Could you check a few things on this model? Use its own coordinates, in mm. Face numbers are marked on the shaded views. A direction names the side the tool comes from. Round coordinates to 2 decimals unless told otherwise and drop trailing zeros. Loops run counter-clockwise (first coordinate to the right, second up) from the corner with the lowest first, then second, coordinate; pieces in that order, holes last. Notation, with made-up numbers: M -6.5,2 L 27.5,2 A22 cw 27.5,41 Z; hole C -2.5,-34.5 d3. An arc over 180 degrees is marked long. Answer in a Markdown table with one row per item.
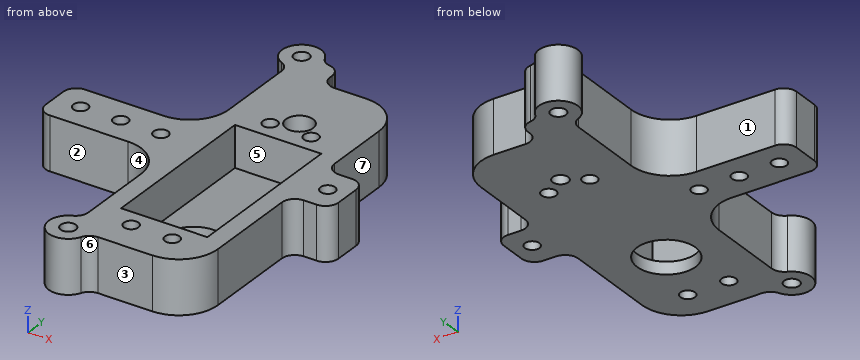
```python
from build123d import *

# Parameters (mm, degrees)
SKETCH1_W               = 31.75
SKETCH1_H               = 12.7
SKETCH1_W_2             = 30
SKETCH1_H_2             = 7
BOSS_EXTRUDE1_DEPTH     = 13
SKETCH4_R               = 1.778
CUT_EXTRUDE3_DEPTH      = 14
SKETCH5_W               = 21
SKETCH5_H               = 41
CUT_EXTRUDE4_DEPTH      = 10
SKETCH6_R               = 7.112
CUT_EXTRUDE5_DEPTH      = 4
SKETCH7_W               = 31.75
SKETCH7_H               = 12.7
CUT_EXTRUDE6_DEPTH      = 6.35
SKETCH10_R              = 1.905
CUT_EXTRUDE8_DEPTH      = 14
SKETCH11_R              = 3.302
CUT_EXTRUDE9_DEPTH      = 9.525
SKETCH13_W              = 9.525
SKETCH13_H              = 12.7
SKETCH13_R              = 1.778
BOSS_EXTRUDE2_DEPTH     = 13
BOSS_EXTRUDE3_DEPTH     = 13
SKETCH18_R              = 1.8415
CUT_EXTRUDE10_DEPTH     = 14
FILLET1_R               = 9.525
FILLET2_R               = 3.175
SKETCH19_W              = 22.225
SKETCH19_H              = 12.7
BOSS_EXTRUDE4_DEPTH     = 7.62
SKETCH8_R               = 1.778
CUT_EXTRUDE7_DEPTH      = 7.35
CUT_EXTRUDE7_DEPTH_BACK = 17.78
FILLET3_R               = 3.175


with BuildPart() as part:
    # Sketch1 → Boss-Extrude1 (new body)
    with BuildSketch(Plane.XY):
        Polygon((31.75, 12.7), (31.75, 0), (31.75, -28.65), (61.75, -28.65), (61.75, 0), (61.75, 12.7), (61.75, 41.35), (31.75, 41.35), align=None)
        with Locations((15.875, 6.35)):
            Rectangle(SKETCH1_W, SKETCH1_H)
        with Locations((46.75, -32.15)):
            Rectangle(SKETCH1_W_2, SKETCH1_H_2)
    extrude(amount=BOSS_EXTRUDE1_DEPTH)

    # Sketch4 → Cut-Extrude3 (cut, through all)
    with BuildSketch(Plane.XY.offset(13)):
        with Locations((41.75, 22.199999832)):
            Circle(SKETCH4_R)
        with Locations((51.75, 22.199999832)):
            Circle(SKETCH4_R)
        with Locations((41.75, -27.800000168)):
            Circle(SKETCH4_R)
        with Locations((51.75, -27.800000168)):
            Circle(SKETCH4_R)
    extrude(amount=-CUT_EXTRUDE3_DEPTH, mode=Mode.SUBTRACT)

    # Sketch5 → Cut-Extrude4 (cut)
    with BuildSketch(Plane.XY.offset(13)):
        with Locations((46.75, -2.800000024)):
            Rectangle(SKETCH5_W, SKETCH5_H)
    extrude(amount=-CUT_EXTRUDE4_DEPTH, mode=Mode.SUBTRACT)

    # Sketch6 → Cut-Extrude5 (cut, through all)
    with BuildSketch(Plane.XY.offset(3)):
        with Locations((46.75, -12.700000168)):
            Circle(SKETCH6_R)
    extrude(amount=-CUT_EXTRUDE5_DEPTH, mode=Mode.SUBTRACT)

    # Sketch7 → Cut-Extrude6 (cut)
    with BuildSketch(Plane(origin=(0, 0, 0), x_dir=(-1, 0, 0), z_dir=(0, 0, -1))):
        with Locations((-15.875, 6.35)):
            Rectangle(SKETCH7_W, SKETCH7_H)
    extrude(amount=-CUT_EXTRUDE6_DEPTH, mode=Mode.SUBTRACT)

    # Sketch10 → Cut-Extrude8 (cut, through all)
    with BuildSketch(Plane(origin=(0, 0, 0), x_dir=(-1, 0, 0), z_dir=(0, 0, -1))):
        with Locations((-46.75, 25.4)):
            Circle(SKETCH10_R)
    extrude(amount=-CUT_EXTRUDE8_DEPTH, mode=Mode.SUBTRACT)

    # Sketch11 → Cut-Extrude9 (cut)
    with BuildSketch(Plane.XY.offset(13)):
        with Locations((46.75, 25.4)):
            Circle(SKETCH11_R)
    extrude(amount=-CUT_EXTRUDE9_DEPTH, mode=Mode.SUBTRACT)

    # Sketch13 → Boss-Extrude2 (add)
    with BuildSketch(Plane.XY.offset(13)):
        with Locations((66.5125, 6.35)):
            Rectangle(SKETCH13_W, SKETCH13_H)
        with Locations((66.5125, 6.35)):
            Circle(SKETCH13_R, mode=Mode.SUBTRACT)
    extrude(amount=-BOSS_EXTRUDE2_DEPTH)

    # Sketch17 → Boss-Extrude3 (add)
    with BuildSketch(Plane.XY.offset(13)):
        with BuildLine():
            ThreePointArc((36.5125, 48.359214074), (28.382403955, 51.726810119), (31.75, 43.596714074))
            Line((31.75, 43.596714074), (31.75, 48.359214074))
            Line((31.75, 48.359214074), (36.5125, 48.359214074))
        make_face()
        with BuildLine():
            Line((31.75, 48.359214074), (31.75, 43.596714074))
            ThreePointArc((31.75, 43.596714074), (35.117596045, 44.991618029), (36.5125, 48.359214074))
            Line((36.5125, 48.359214074), (31.75, 48.359214074))
        make_face()
        with BuildLine():
            Line((31.75, 43.596714074), (31.75, 41.35))
            Line((31.75, 41.35), (41.275, 41.35))
            Line((41.275, 41.35), (41.275, 48.359214074))
            Line((41.275, 48.359214074), (36.5125, 48.359214074))
            ThreePointArc((36.5125, 48.359214074), (35.117596045, 44.991618029), (31.75, 43.596714074))
        make_face()
        with BuildLine():
            Line((31.75, -35.65), (36.5125, -35.65))
            ThreePointArc((36.5125, -35.65), (35.117596045, -32.282403955), (31.75, -30.8875))
            Line((31.75, -30.8875), (31.75, -35.65))
        make_face()
        with BuildLine():
            ThreePointArc((31.75, -30.8875), (28.382403955, -39.017596045), (36.5125, -35.65))
            Line((36.5125, -35.65), (31.75, -35.65))
            Line((31.75, -35.65), (31.75, -30.8875))
        make_face()
    extrude(amount=-BOSS_EXTRUDE3_DEPTH)

    # Sketch18 → Cut-Extrude10 (cut, through all)
    with BuildSketch(Plane.XY.offset(13)):
        with Locations((31.75, -35.65)):
            Circle(SKETCH18_R)
        with Locations((31.75, 48.359214074)):
            Circle(SKETCH18_R)
    extrude(amount=-CUT_EXTRUDE10_DEPTH, mode=Mode.SUBTRACT)

    # Fillet1
    fillet1_edges = [part.edges().sort_by_distance(p)[0] for p in [
        (31.75, 0, 9.675),
        (31.75, 12.7, 9.675),
        (61.75, 41.35, 6.5),
        (61.75, -35.65, 6.5),
    ]]
    fillet(fillet1_edges, radius=FILLET1_R)

    # Fillet2
    fillet2_edges = [part.edges().sort_by_distance(p)[0] for p in [
        (71.275, 0, 6.5),
        (71.275, 12.7, 6.5),
        (61.75, 12.7, 6.5),
        (61.75, 0, 6.5),
        (31.75, -30.8875, 6.5),
        (36.5125, -35.65, 6.5),
        (31.75, 43.596714074, 6.5),
        (41.275, 41.35, 6.5),
        (36.5125, 48.359214074, 6.5),
    ]]
    fillet(fillet2_edges, radius=FILLET2_R)

    # Sketch19 → Boss-Extrude4 (add)
    with BuildSketch(Plane.XY):
        with BuildLine():
            ThreePointArc((31.75, -9.525), (28.960192091, -2.789807909), (22.225, 0))
            Line((22.225, 0), (22.225, 12.7))
            ThreePointArc((22.225, 12.7), (28.960192091, 15.489807909), (31.75, 22.225))
            Line((31.75, 22.225), (31.75, -9.525))
        make_face()
        with Locations((11.1125, 6.35)):
            Rectangle(SKETCH19_W, SKETCH19_H)
    extrude(amount=BOSS_EXTRUDE4_DEPTH)

    # Sketch8 → Cut-Extrude7 (cut, two sides)
    with BuildSketch(Plane(origin=(0, 0, 6.35), x_dir=(-1, 0, 0), z_dir=(0, 0, -1))) as cut_extrude7_sk:
        with Locations((-6.35, 6.35)):
            Circle(SKETCH8_R)
        with Locations((-25.908, 6.35)):
            Circle(SKETCH8_R)
        with Locations((-16.129, 6.35)):
            Circle(SKETCH8_R)
    extrude(amount=CUT_EXTRUDE7_DEPTH, mode=Mode.SUBTRACT)
    extrude(cut_extrude7_sk.sketch, amount=-CUT_EXTRUDE7_DEPTH_BACK, mode=Mode.SUBTRACT)

    # Fillet3
    fillet3_edges = [part.edges().sort_by_distance(p)[0] for p in [
        (41.275, 48.359214074, 6.5),
        (0, 12.7, 6.5),
        (0, 0, 6.5),
    ]]
    fillet(fillet3_edges, radius=FILLET3_R)


solid = part.part
```
1) If we mould it in two halves opening along Y, with no side actions, what happens to the marked faces 5, 6 and 7? For each: released by +Y, released by -Y, zero draft, split by the parting line, or undercut.
Computed:
| item | result |
|---|---|
| face 5 | undercut |
| face 6 | released by -Y |
| face 7 | zero draft |
2) I want a section at D-D, the plane x = 55.5. Please give me the cut outline in (y, z).
Computed:
| item | result |
|---|---|
| outline | M -35.07,0 L 40.77,0 L 40.77,13 L 17.7,13 L 17.7,3 L -23.3,3 L -23.3,13 L -35.07,13 Z |
3) I need wall thicknesses on line 1 (Y direction, x = 6.35, z = 8); line 2 (X direction, y = 7.5, z = 1.5) (3 decimals); line 3 (X direction, y = -16.5, z = 12). Which ranges of each line are inside material? Lowest first, please.
Computed:
| item | result |
|---|---|
| line 1 | y = 0 to 4.57, 8.13 to 12.7 |
| line 2 | x = 0 to 4.994, 7.706 to 14.773, 17.485 to 24.552, 27.264 to 65.156, 67.869 to 71.275 |
| line 3 | x = 31.75 to 36.25, 57.25 to 61.75 |
4) Which directions (+Z, -Z, +X, -X, +Y, -Y) give clear straight access to the entire face, cutting with the end or side of a thin tool? Please do the marked faces 1, 2, 3 and 4.
Computed:
| item | result |
|---|---|
| face 1 | +Z, -Z, -X, +Y |
| face 2 | +Z, -Z, -X, -Y |
| face 3 | +Z, -Z, +X, -Y |
| face 4 | +Z, -Z, -X |
5) I want a section at B-B, the plane x = 46.75. Please give me the cut outline in (y, z) (3 decimals).
Computed:
| item | result |
|---|---|
| outline | M -35.65,0 L -19.812,0 L -19.812,3 L -23.3,3 L -23.3,13 L -35.65,13 Z; M -5.588,0 L 23.495,0 L 23.495,3.475 L 22.098,3.475 L 22.098,13 L 17.7,13 L 17.7,3 L -5.588,3 Z; M 27.305,0 L 41.35,0 L 41.35,13 L 28.702,13 L 28.702,3.475 L 27.305,3.475 Z |
6) I want a section at C-C, the plane y = -8.5. Please give me the cut outline in (x, z).
Computed:
| item | result |
|---|---|
| outline | M 31.69,0 L 41.01,0 L 41.01,3 L 36.25,3 L 36.25,13 L 31.69,13 Z; M 52.49,0 L 61.75,0 L 61.75,13 L 57.25,13 L 57.25,3 L 52.49,3 Z |
7) Will these pins go through, and if not, where does the flat tip stop? P1, Ø2, axis at x = 16.129, y = 6.35, coming from the +Z side; P2, Ø4, axis at x = 16.5, z = 3.5, coming from the +Y side; P3, Ø0.6, axis at y = 45, z = 4.5, coming from the +X side (3 decimals); P4, Ø5, axis at y = 18.5, z = 10.5, coming from the -X side.
Computed:
| item | result |
|---|---|
| P1 | passes through |
| P2 | stops at y = 12.7 |
| P3 | stops at x = 41.275 |
| P4 | stops at x = 29.43 |
8) I want a section at A-A, the plane x = 6.35. Please give me the cut outline in (y, z).
Computed:
| item | result |
|---|---|
| outline | M 0,0 L 4.57,0 L 4.57,13 L 0,13 Z; M 8.13,0 L 12.7,0 L 12.7,13 L 8.13,13 Z |
